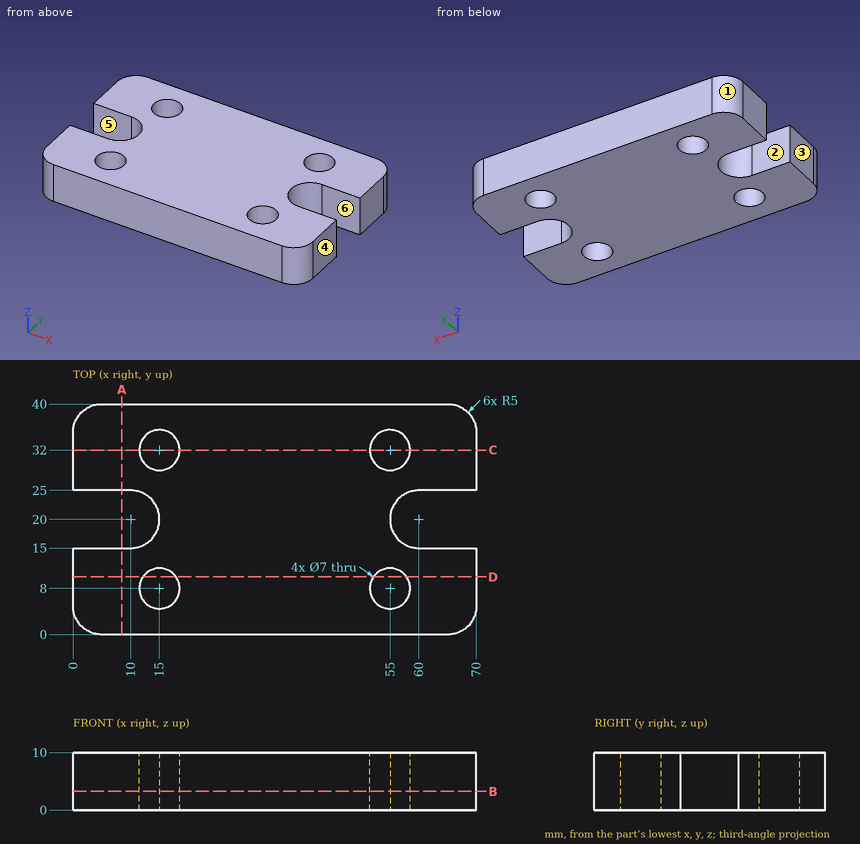
Verification items for this drawing (mm, ordinates from the low corner). A direction names the side the tool comes from. Coordinates: 2 decimals unless noted, no trailing zeros. Write each loop counter-clockwise with the first axis right and the second up, starting at its lowest first coordinate (ties: lowest second). Pieces come first, ordered by that corner, then holes. Notation, with made-up numbers: (-30.5, 61) - (-4.5, 61) arc R26 ccw to (-4.5, 94) - close; hole circle Ø11 at (64, 76). An arc over 180 degrees is marked (long way). One line per question, with ' | ' between items.
Item 1: Sectioned sample at D-D on y = 10. Record the boundary of the cut face in (x, z).
Determined:
outline: (0, 0) - (12.13, 0) - (12.13, 10) - (0, 10) - close; (17.87, 0) - (52.13, 0) - (52.13, 10) - (17.87, 10) - close; (57.87, 0) - (70, 0) - (70, 10) - (57.87, 10) - close
Item 2: Thickness scan on line 1 (X direction, y = 30.5, z = 8); line 2 (X direction, y = 6, z = 8.25); line 3 (Y direction, x = 60, z = 0.5). Record the ranges inside material, lowest first. Write a range as [from, to].
Determined:
line 1: x = [0, 11.84], [18.16, 51.84], [58.16, 70] | line 2: x = [0, 12.13], [17.87, 52.13], [57.87, 70] | line 3: y = [0, 15], [25, 40]
Item 3: Sectioned sample at B-B on z = 3.25. Record the boundary of the cut face in (x, y), plus the area to 3 significant figures.
Determined:
outline: (0, 5) arc R5 ccw to (5, 0) - (65, 0) arc R5 ccw to (70, 5) - (70, 15) - (60, 15) arc R5 cw to (60, 25) - (70, 25) - (70, 35) arc R5 ccw to (65, 40) - (5, 40) arc R5 ccw to (0, 35) - (0, 25) - (10, 25) arc R5 cw to (10, 15) - (0, 15) - close; hole circle Ø7 at (15, 8); hole circle Ø7 at (15, 32); hole circle Ø7 at (55, 8); hole circle Ø7 at (55, 32) | area: 2,350 mm2
Item 4: Mould release check, pull along Y, two halves, no side actions. Record for the marked faces 1, 2 and 3: pulls with the +Y half, pulls with the -Y half, needs draft (parallel to the pull), parting line crosses it, or undercut.
Determined:
face 1: pulls with the +Y half | face 2: undercut | face 3: needs draft
Item 5: Sectioned sample at A-A on x = 8.5. Record the boundary of the cut face in (y, z).
Determined:
outline: (0, 0) - (15, 0) - (15, 10) - (0, 10) - close; (25, 0) - (40, 0) - (40, 10) - (25, 10) - close
Item 6: Sectioned sample at C-C on y = 32. Record the boundary of the cut face in (x, z), plus the area to 3 significant figures.
Determined:
outline: (0, 0) - (11.5, 0) - (11.5, 10) - (0, 10) - close; (18.5, 0) - (51.5, 0) - (51.5, 10) - (18.5, 10) - close; (58.5, 0) - (70, 0) - (70, 10) - (58.5, 10) - close | area: 560 mm2
Item 7: Access from +Z, -Z, +X, -X, +Y, -Y to the whole of each face (thin tool, end or side, straight path). Record for the marked faces 4, 5 and 6.
Determined:
face 4: +Z, -Z, +X, +Y, -Y | face 5: +Z, -Z, -X | face 6: +Z, -Z, +X
Item 8: Gauge pin test, flat ends, axial feed: P1, Ø12, axis at x = 18.5, y = 28, coming from the -Z side; P2, Ø4, axis at x = 55, y = 32, coming from the -Z side. Record the tip position at first contact, or that the pin passes through.
Determined:
P1: stops at z = 0 | P2: passes through
